from build123d import *

# Parameters (mm, degrees)
F1_DEPTH = 2.9
F2_R     = 1.75
F2_R_2   = 11.05
F3_DEPTH = 2.9
F4_R     = 2.9
F7_DEPTH = 2.5


with BuildPart() as f1:
    # F0 (on Front) → F1 (new body)
    with BuildSketch(Plane.XZ):
        Polygon((-25, 48.3), (-25, 0), (25, 0), (25, 48.3), (20, 53.3), (-20, 53.3), align=None)
        with BuildLine():
            ThreePointArc((-19.32, 44.3), (-17.2, 46.42), (-15.08, 44.3))
            Line((-15.08, 44.3), (-15.08, 14.34))
            ThreePointArc((-15.08, 14.34), (-17.2, 12.22), (-19.32, 14.34))
            Line((-19.32, 14.34), (-19.32, 44.3))
        make_face(mode=Mode.SUBTRACT)
        with BuildLine():
            ThreePointArc((15.08, 44.3), (17.2, 46.42), (19.32, 44.3))
            Line((19.32, 44.3), (19.32, 14.34))
            ThreePointArc((19.32, 14.34), (17.2, 12.22), (15.08, 14.34))
            Line((15.08, 14.34), (15.08, 44.3))
        make_face(mode=Mode.SUBTRACT)
    extrude(amount=F1_DEPTH)

    # F2 (on Top) → F3 (join)
    with BuildSketch(Plane.XY):
        Polygon((25, 0), (-25, 0), (-25, -43.6), (-20, -48.6), (20, -48.6), (25, -43.6), align=None)
        with Locations((-17.2, -44.7)):
            Circle(F2_R, mode=Mode.SUBTRACT)
        with Locations((17.2, -44.7)):
            Circle(F2_R, mode=Mode.SUBTRACT)
        with Locations((0, -27.65)):
            Circle(F2_R_2, mode=Mode.SUBTRACT)
        with Locations((-17.2, -13.7)):
            Circle(F2_R, mode=Mode.SUBTRACT)
        with Locations((17.2, -13.7)):
            Circle(F2_R, mode=Mode.SUBTRACT)
    extrude(amount=F3_DEPTH)

    # F4
    f4_edges = [f1.edges().sort_by_distance(p)[0] for p in [
        (0, -2.9, 2.9),
        (0, 0, 0),
    ]]
    fillet(f4_edges, radius=F4_R)

    # F6 (on offset) → F7 (join)
    with BuildSketch(Plane.YZ.offset(25)):
        with BuildLine():
            Line((-3.700844, 19.396721), (-24.406105, 3.799366))
            ThreePointArc((-24.406105, 3.799366), (-24.579436, 3.241385), (-24.105261, 2.9))
            Line((-24.105261, 2.9), (-6.861522, 2.9))
            Line((-6.861522, 2.9), (-2.9, 6.861522))
            Line((-2.9, 6.861522), (-2.9, 18.997355))
            ThreePointArc((-2.9, 18.997355), (-3.176865, 19.444805), (-3.700844, 19.396721))
        make_face()
    extrude(amount=-F7_DEPTH)

    # F8: F1 across plane


with BuildPart() as f1_1:
    add(f1.part)
    add(f1.part.mirror(Plane.YZ))


solid = f1_1.part
Could you check a few things on this model? Use its own coordinates, in mm. A direction names the side the tool comes from. Give positions to 0.01 mm unless a question says otherwise; leave off trailing zeros. Order: outer loops, then holes, each group sorted by start corner. A loop starts at its lowest first (then second) coordinate and runs counter-clockwise, first axis right, second up.
1. Suppose I cut it at D-D (y = -27.65). List the corners of the cut face in (x, z) for me, plus the area to 3 significant figures.
2. Suppose I cut it at A-A (x = 0). List the corners of the cut face in (y, z) for me.
3. Will these pins go through, and if not, where does the flat tip stop? P1, Ø24, axis at x = 12, z = 37, coming from the -Y side; P2, Ø4, axis at x = 17.2, y = -13.7, coming from the +Z side.
4. For faces 5 (the flat face through (0, -1, 53.3)), 6 (the flat face through (22.5, -11, 9)), 7 (the cylindrical face through (17.15, -1.43, 46.42)), which set-ups out of +Z, -Z, +X, -X, +Y, -Y let a thin tool reach every point of the face, with its end or its side?
5. I need wall thicknesses on L1, parallel to X at y = -2, z = 40.5; L2, parallel to Y at x = 17.2, z = 1.6; L3, parallel to X at y = -44, z = 1. Which ranges of each line are inside material? Lowest first, please.
6. Suppose I cut it at C-C (z = 40). List the corners of the cut face in (x, y) for me.
7. Suppose I cut it at B-B (y = -44.7). List the corners of the cut face in (x, z) for me, plus the area to 3 significant figures.
8. We'd pull the mould along Z, two halves only. Please class faces 1 (the flat face through (23.77, -4.91, 4.85)), 2 (the cylindrical face through (-15.531, -44.174, 1.43)), 3 (the flat face through (22.5, -1.4, 50.8)), 4 (the flat face through (-15.08, -1, 30)): pulls with the +Z half, pulls with the -Z half, needs draft (parallel to the pull), parting line crosses it, or undercut.
Solved:
1. outline: (-25, 0) - (-11.05, 0) - (-11.05, 2.9) - (-25, 2.9) - close; (11.05, 0) - (25, 0) - (25, 2.9) - (11.05, 2.9) - close
1. area: 80.9 mm2
2. outline: (-48.6, 0) - (-38.7, 0) - (-38.7, 2.9) - (-48.6, 2.9) - close; (-16.6, 0) - (-2.9, 0) arc R2.9 ccw to (0, 2.9) - (0, 53.3) - (-2.9, 53.3) - (-2.9, 5.8) arc R2.9 cw to (-5.8, 2.9) - (-16.6, 2.9) - close
3. P1: stops at y = -2.9
3. P2: stops at z = 2.9
4. face 5: +Z, +X, -X, +Y, -Y
4. face 6: +Z, -Y
4. face 7: +Y, -Y
5. L1: x = -25 to -19.32, -15.08 to 15.08, 19.32 to 25
5. L2: y = -48.6 to -46.45, -42.95 to -15.45, -11.95 to -0.31
5. L3: x = -24.6 to -18.8, -15.6 to 15.6, 18.8 to 24.6
6. outline: (-25, -2.9) - (-19.32, -2.9) - (-19.32, 0) - (-25, 0) - close; (-15.08, -2.9) - (15.08, -2.9) - (15.08, 0) - (-15.08, 0) - close; (19.32, -2.9) - (25, -2.9) - (25, 0) - (19.32, 0) - close
7. outline: (-23.9, 0) - (-18.95, 0) - (-18.95, 2.9) - (-23.9, 2.9) - close; (-15.45, 0) - (15.45, 0) - (15.45, 2.9) - (-15.45, 2.9) - close; (18.95, 0) - (23.9, 0) - (23.9, 2.9) - (18.95, 2.9) - close
7. area: 118 mm2
8. face 1: undercut
8. face 2: needs draft
8. face 3: pulls with the +Z half
8. face 4: undercut
